from build123d import *

# Parameters (mm, degrees)
SKETCH1_R           = 1.5
SKETCH1_R_2         = 2
BOSS_EXTRUDE1_DEPTH = 3
FILLET1_R           = 3


with BuildPart() as part:
    # Sketch1 → Boss-Extrude1 (new body)
    with BuildSketch(Plane(origin=(0, 0, 0), x_dir=(1, 0, 0), z_dir=(0, 1, 0))):
        with BuildLine():
            ThreePointArc((3.16227766, 1.5), (-3.5, 0), (3.16227766, -1.5))
            Line((3.16227766, -1.5), (27.83772234, -1.5))
            ThreePointArc((27.83772234, -1.5), (34.5, 0), (27.83772234, 1.5))
            Line((27.83772234, 1.5), (3.16227766, 1.5))
        make_face()
        with Locations(Location((0, 0, 0), (0, 0, 270))):
            Circle(SKETCH1_R, mode=Mode.SUBTRACT)
        with Locations(Location((31, 0, 0), (0, 0, 270))):
            Circle(SKETCH1_R_2, mode=Mode.SUBTRACT)
    extrude(amount=BOSS_EXTRUDE1_DEPTH)

    # Fillet1
    fillet1_edges = [part.edges().sort_by_distance(p)[0] for p in [
        (27.83772234, 1.5, 1.5),
        (3.16227766, 1.5, 1.5),
        (3.16227766, 1.5, -1.5),
        (27.83772234, 1.5, -1.5),
    ]]
    fillet(fillet1_edges, radius=FILLET1_R)


solid = part.part
Design review of the part built by this model. Coordinates are the model's own, in mm. A direction names the side the tool comes from. Give positions to 0.01 mm unless a question says otherwise; leave off trailing zeros. Write each loop counter-clockwise with the first axis right and the second up, starting at its lowest first coordinate (ties: lowest second). Pieces come first, ordered by that corner, then holes. Notation, with made-up numbers: M -24.5,-12 L 12.5,-12 A23 cw 12.5,12 Z; hole C 8,-1.5 d2. An arc over 180 degrees is marked long. Return JSON: item names as keys, results as strings. Group by question number.
Item 1: Take a section at D-D (x = 31). Give the boundary of the cut face in (y, z).
Item 2: Clearance check with flat-ended pins moving along their axes: pin 1 Ø0.9 at (x, y) = (14.5, 1) entering from -Z; pin 2 Ø1.5 at (x, y) = (10.5, 1.5) entering from +Z. State where each tip first meets the part, or that it passes through.
Item 3: Take a section at B-B (z = 0). Give the boundary of the cut face in (x, y), plus the area to 3 significant figures.
Item 4: Wall thickness on line 1 along X through (y, z) = (1.65, 0); line 2 along X through (y, z) = (2.75, 2.75); line 3 along X through (y, z) = (0.45, -0.75): over which ranges is each line inside the solid? List them lowest first.
Item 5: Take a section at A-A (y = 1.15). Give the boundary of the cut face in (x, z).
Item 6: The part is to be moulded in two halves that separate along X. For faces 4 (the flat face through (16, 1, -1.5)), 5 (the flat face through (11, 0, 0)), 6 (the cylindrical face through (0.45, 1.48, 1.43)), say which applies: pulls with the +X half, pulls with the -X half, needs draft (parallel to the pull), parting line crosses it, or undercut.
Item 7: Tool access review of faces 1 (the cylindrical face through (27.471, 1.521, -1.734)), 2 (the cylindrical face through (27.471, 1.521, 1.734)), 3 (the flat face through (11, 3, 0)): name each direction out of +Z, -Z, +X, -X, +Y, -Y from which nothing blocks a thin tool from reaching the whole face with its end or side.
Item 8: Take a section at C-C (x = 0). Give the boundary of the cut face in (y, z).
Return value:
{
 "1": {"outline": "M 0,-3.5 L 3,-3.5 L 3,-2 L 0,-2 Z; M 0,2 L 3,2 L 3,3.5 L 0,3.5 Z"},
 "2": {"pin 1": "stops at z = -1.5", "pin 2": "stops at z = 1.5"},
 "3": {"outline": "M -3.5,0 L -1.5,0 L -1.5,3 L -3.5,3 Z; M 1.5,0 L 29,0 L 29,3 L 1.5,3 Z; M 33,0 L 34.5,0 L 34.5,3 L 33,3 Z", "area": "93.0 mm2"},
 "4": {"line 1": "x = -3.5 to -1.5, 1.5 to 29, 33 to 34.5", "line 2": "x = -2.17 to 2.17, 28.83 to 33.17", "line 3": "x = -3.42 to -1.3, 1.3 to 29.15, 32.85 to 34.42"},
 "5": {"outline": "M 2.53,-2.42 A3 cw 4.69,-1.5 L 26.31,-1.5 A3 cw 28.47,-2.42 A3.5 ccw long 28.47,2.42 A3 cw 26.31,1.5 L 4.69,1.5 A3 cw 2.53,2.42 A3.5 ccw long Z; hole C 0,0 d3; hole C 31,0 d4"},
 "6": {"face 4": "undercut", "face 5": "needs draft", "face 6": "undercut"},
 "7": {"face 1": "-Z, +Y, -Y", "face 2": "+Z, +Y, -Y", "face 3": "+Z, -Z, +X, -X, +Y"},
 "8": {"outline": "M 0,-3.5 L 3,-3.5 L 3,-1.5 L 0,-1.5 Z; M 0,1.5 L 3,1.5 L 3,3.5 L 0,3.5 Z"}
}
